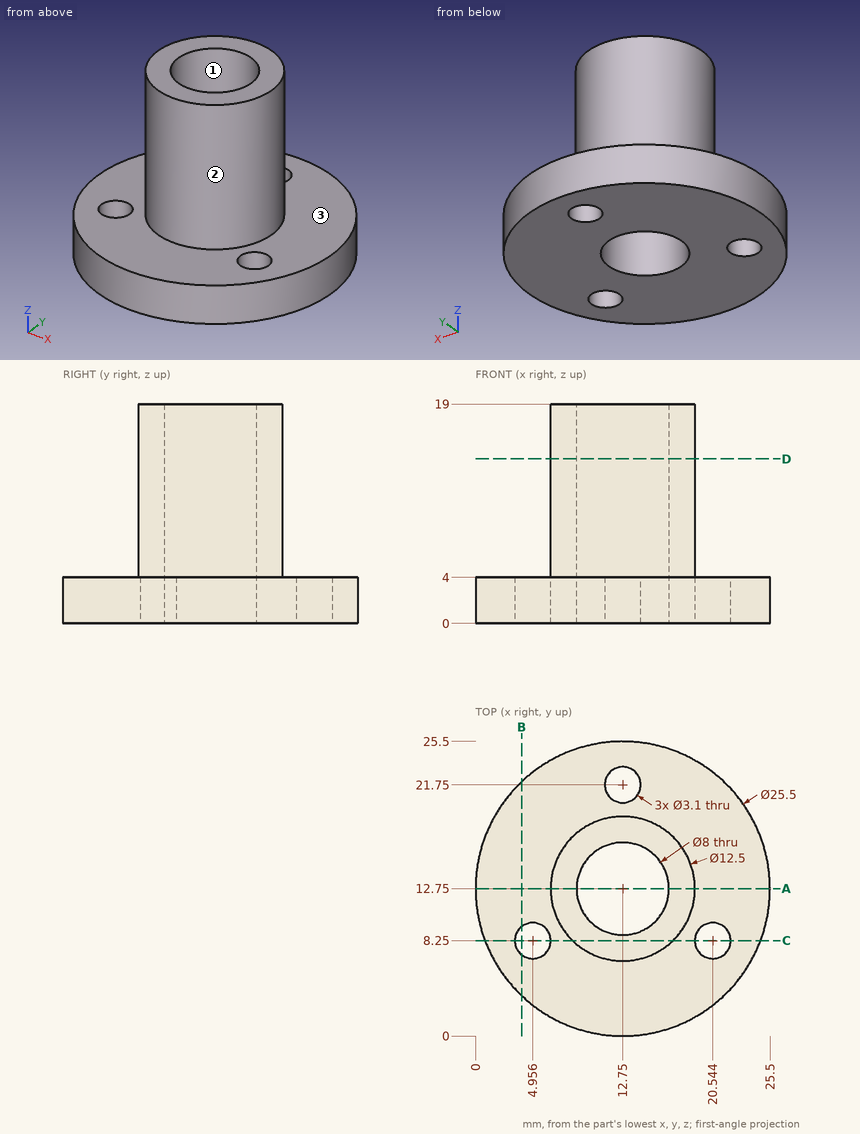
Input: dimensioned drawing with shaded views. Units: mm. Origin: part minimum x, y, z. Round coordinates to 2 decimals unless told otherwise and drop trailing zeros. Loops run counter-clockwise (first coordinate to the right, second up) from the corner with the lowest first, then second, coordinate; pieces in that order, holes last. Notation, with made-up numbers: M 55,12.25 L 110,12.25 A8 ccw 110,25.25 Z; hole C 64,-5.5 d7. An arc over 180 degrees is marked long. Return JSON: item names as keys, results as strings. Group by question number.
1. Section query A-A on y = 12.75. Output: boundary loops of the cut face in (x, z), and give its area (4 significant figures).
2. Section query D-D on z = 14.25. Output: boundary loops of the cut face in (x, y).
3. Section query C-C on y = 8.25. Output: boundary loops of the cut face in (x, z).
4. Mould query, pull axis Y, two halves, no side actions, for the marked faces 1, 2 and 3. Classes: released by +Y, released by -Y, zero draft, split by the parting line, or undercut.
5. Section query B-B on x = 4. Output: boundary loops of the cut face in (y, z).
6. Material intervals for line 1 along Y through (x, z) = (12.75, 14.5); line 2 along Z through (x, y) = (17, 5.75), sorted ascending. Write a range as from..to.
7. Pin query (flat end, axial travel): pin 1 (1 mm diameter, centred on x = 13.5, z = 9, fed in from -Y) (3 decimals); pin 2 (5 mm diameter, centred on x = 20.54, y = 8.25, fed in from +Z); pin 3 (6 mm diameter, centred on y = 20.5, z = 5.5, fed in from +X). Return the tip coordinate at first contact, or that it passes through.
Checks:
{
 "1": {"outline": "M 0,0 L 8.75,0 L 8.75,19 L 6.5,19 L 6.5,4 L 0,4 Z; M 16.75,0 L 25.5,0 L 25.5,4 L 19,4 L 19,19 L 16.75,19 Z", "area": "137.5 mm²"},
 "2": {"outline": "C 12.75,12.75 d12.5; hole C 12.75,12.75 d8"},
 "3": {"outline": "M 0.82,0 L 3.41,0 L 3.41,4 L 0.82,4 Z; M 6.51,0 L 18.99,0 L 18.99,4 L 17.09,4 L 17.09,19 L 8.41,19 L 8.41,4 L 6.51,4 Z; M 22.09,0 L 24.68,0 L 24.68,4 L 22.09,4 Z"},
 "4": {"face 1": "undercut", "face 2": "split by the parting line", "face 3": "zero draft"},
 "5": {"outline": "M 3.48,0 L 7.03,0 L 7.03,4 L 3.48,4 Z; M 9.47,0 L 22.02,0 L 22.02,4 L 9.47,4 Z"},
 "6": {"line 1": "y = 6.5..8.75, 16.75..19", "line 2": "z = 0..4"},
 "7": {"pin 1": "stops at y = 6.505", "pin 2": "stops at z = 4", "pin 3": "stops at x = 24.41"}
}
